Job drawing, mm, ordinate dimensions from the low corner. One solid piece. Give positions to 0.01 mm unless a question says otherwise; leave off trailing zeros. One line per question, with ' | ' between items.
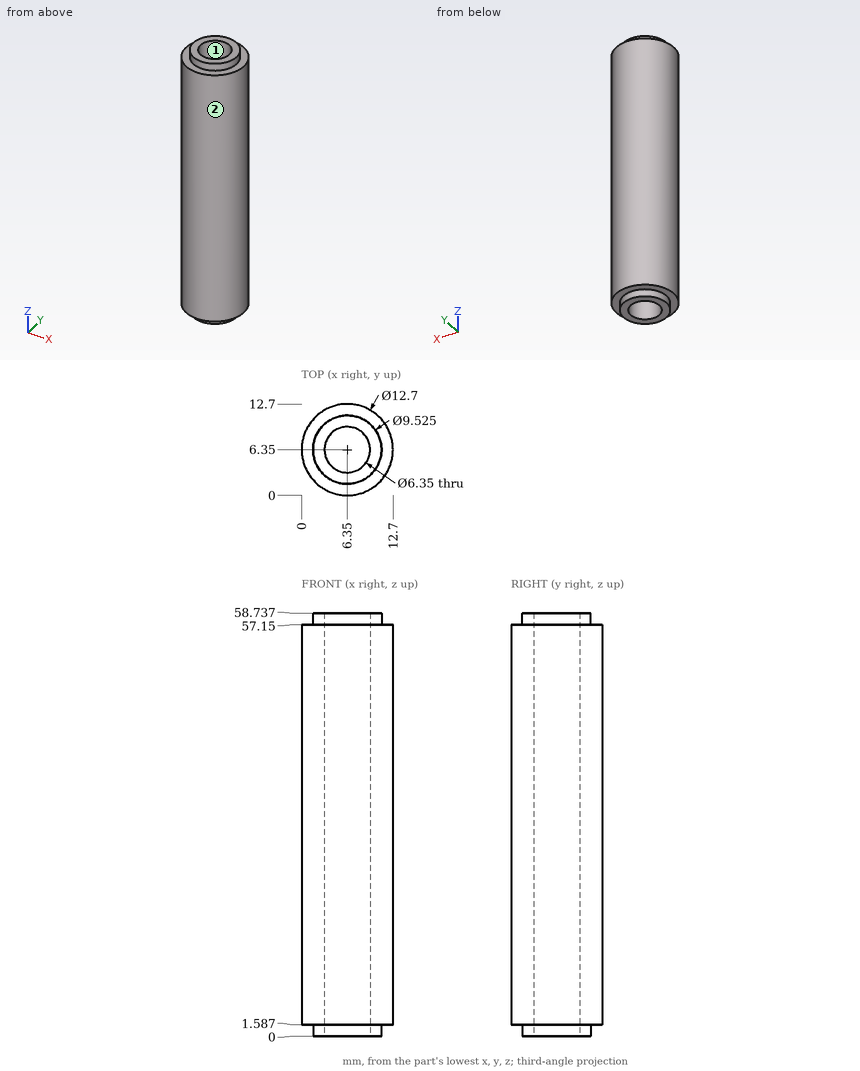
Item 1: Drill centre lines: line 1 along Y through (x, z) = (6.35, 42) (1 decimal); line 2 along X through (y, z) = (5.5, 54.5); line 3 along X through (y, z) = (9, 42) (1 decimal). Where is each one in solid material? Low to high. Write a range as [from, to].
Conclusion:
line 1: [0, 3.2], [9.5, 12.7] | line 2: [0.06, 3.29], [9.41, 12.64] | line 3: [0.6, 4.6], [8.1, 12.1]
Item 2: Mould opens along X. For the marked faces 1 and 2 say: pulls with the +X half, pulls with the -X half, needs draft (parallel to the pull), parting line crosses it, or undercut.
Conclusion:
face 1: undercut | face 2: parting line crosses it
Item 3: Drop flat-ended pins along their axis: P1, Ø5, axis at x = 2.5, z = 13.5, coming from the -Y side (1 decimal); P2, Ø5.5, axis at x = 6.35, y = 6.35, coming from the +Z side; P3, Ø1.5, axis at x = 5, z = 26.5, coming from the +Y side; P4, Ø1, axis at y = 9.5, z = 11.5, coming from the -X side. Give the stop position or say it passes through.
Conclusion:
P1: y = 0.1 | P2: through | P3: y = 12.67 | P4: x = 0.58
